Check sheet for the modelled part. Datum: model origin and axes. Units: mm. A direction names the side the tool comes from. Round coordinates to 2 decimals unless told otherwise and drop trailing zeros. Write each loop counter-clockwise with the first axis right and the second up, starting at its lowest first coordinate (ties: lowest second). Pieces come first, ordered by that corner, then holes. Notation, with made-up numbers: (-1.5, -7) -> (56.5, -7) arc R21 ccw to (56.5, 23) -> close; hole circle Ø5 at (-9.5, -32.75). An arc over 180 degrees is marked (long way). Answer as a JSON object with one key per item and string values. Group by question number.
```python
from build123d import *

# Parameters (mm, degrees)
BOSS_EXTRUDE1_DEPTH = 20
BOSS_EXTRUDE2_DEPTH = 2


with BuildPart() as part:
    # Sketch1 → Boss-Extrude1 (new body)
    with BuildSketch(Plane(origin=(0, 0, 0), x_dir=(1, 0, 0), z_dir=(0, 1, 0))):
        with BuildLine():
            Line((-1.5, -13.064168554), (-1.5, -13.919410907))
            ThreePointArc((-1.5, -13.919410907), (0, 14), (1.5, -13.919410907))
            Line((1.5, -13.919410907), (1.5, -13.064168554))
            ThreePointArc((1.5, -13.064168554), (0, 13.15), (-1.5, -13.064168554))
        make_face()
    extrude(amount=BOSS_EXTRUDE1_DEPTH)

    # Sketch2 → Boss-Extrude2 (add)
    with BuildSketch(Plane(origin=(0, 20, 0), x_dir=(1, 0, 0), z_dir=(0, 1, 0))):
        with BuildLine():
            Line((-1.5, -13.064168554), (-1.5, -16.888391582))
            ThreePointArc((-1.5, -16.888391582), (0, 16.954874527), (1.5, -16.888391582))
            Line((1.5, -16.888391582), (1.5, -13.064168554))
            ThreePointArc((1.5, -13.064168554), (0, 13.15), (-1.5, -13.064168554))
        make_face()
    extrude(amount=BOSS_EXTRUDE2_DEPTH)


solid = part.part
```
(1) Section check C-C on x = 0. Record the cut outline in (y, z), then the cut area to 3 significant figures.
(2) Release check for a two-part mould opening along X. For faces 1 (the cylindrical face through (-0.72, 20.99, -16.94)), 2 (the flat face through (1.5, 13.4, 13.7)), 3 (the flat face through (-4.9, 22, 12.4)) record: pulls with the +X half, pulls with the -X half, needs draft (parallel to the pull), parting line crosses it, or undercut.
(3) Scan lines: line 1 along X through (y, z) = (8.5, 0); line 2 along Z through (x, y) = (0, 5); line 3 along Z through (x, y) = (-6.5, 14.25). Record each from-to range of solid material in increasing order.
(4) Section check B-B on x = -6. Record the cut outline in (y, z), then the cut area to 3 significant figures.
(5) Section check A-A on z = 0. Record the cut outline in (x, y).
(6) Section check D-D on y = 5. Record the cut outline in (x, z).
(7) Access from +Z, -Z, +X, -X, +Y, -Y to the whole of each face (thin tool, end or side, straight path). Record for faces 4 (the cylindrical face through (-0.595, 9.86, -13.987)), 5 (the cylindrical face through (0.56, 10.85, -13.14)), 6 (the flat face through (-1.5, 13.4, 13.7)).
(8) Go/stop test with flat-tipped pins: pin 1 Ø1.9 at (y, z) = (10.5, 15.5) entering from -X; pin 2 Ø10 at (x, y) = (10.5, 5.5) entering from -Z; pin 3 Ø4 at (y, z) = (16.5, -6.5) entering from -X; pin 4 Ø5 at (y, z) = (14.5, 10) entering from -X. Record where each tip stops, or that it passes through.
Data:
{
 "1": {"outline": "(0, -14) -> (20, -14) -> (20, -16.95) -> (22, -16.95) -> (22, -13.15) -> (0, -13.15) -> close", "area": "24.6 mm²"},
 "2": {"face 1": "parting line crosses it", "face 2": "undercut", "face 3": "needs draft"},
 "3": {"line 1": "x = -14 to -13.15, 13.15 to 14", "line 2": "z = -14 to -13.15", "line 3": "z = -12.4 to -11.43, 11.43 to 12.4"},
 "4": {"outline": "(0, -12.65) -> (20, -12.65) -> (20, -15.86) -> (22, -15.86) -> (22, -11.7) -> (0, -11.7) -> close; (0, 11.7) -> (22, 11.7) -> (22, 15.86) -> (20, 15.86) -> (20, 12.65) -> (0, 12.65) -> close", "area": "54.5 mm²"},
 "5": {"outline": "(-16.95, 20) -> (-14, 20) -> (-14, 0) -> (-13.15, 0) -> (-13.15, 22) -> (-16.95, 22) -> close; (13.15, 0) -> (14, 0) -> (14, 20) -> (16.95, 20) -> (16.95, 22) -> (13.15, 22) -> close"},
 "6": {"outline": "(-1.5, 13.06) -> (-1.5, 13.92) arc R14 ccw (long way) to (1.5, 13.92) -> (1.5, 13.06) arc R13.15 cw (long way) to start"},
 "7": {"face 4": "-Y", "face 5": "+Y, -Y", "face 6": "+Z, +Y, -Y"},
 "8": {"pin 1": "passes through", "pin 2": "stops at z = -12.87", "pin 3": "stops at x = -13.26", "pin 4": "stops at x = -11.82"}
}
